from build123d import *

# Parameters (mm, degrees)
SKETCH1_W           = 20
SKETCH1_H           = 16
SKETCH1_R           = 3
SKETCH1_R_2         = 1.5
BOSS_EXTRUDE1_DEPTH = 11.5
CUT_EXTRUDE1_DEPTH  = 17
SKETCH3_R           = 1.5
SKETCH3_R_2         = 0.775
CUT_EXTRUDE2_DEPTH  = 4
CHAMFER1_SIZE       = 0.3


with BuildPart() as part:
    # Sketch1 → Boss-Extrude1 (new body)
    with BuildSketch(Plane(origin=(0, 0, 0), x_dir=(1, 0, 0), z_dir=(0, 1, 0))):
        with Locations((10, 8)):
            Rectangle(SKETCH1_W, SKETCH1_H)
        with Locations((15.5, 8)):
            Circle(SKETCH1_R, mode=Mode.SUBTRACT)
        with Locations((2.5, 8)):
            Circle(SKETCH1_R_2, mode=Mode.SUBTRACT)
    extrude(amount=BOSS_EXTRUDE1_DEPTH)

    # Sketch2 → Cut-Extrude1 (cut, through all)
    with BuildSketch(Plane.XY):
        with BuildLine():
            Line((5.516608474, 4.5), (11.483391526, 4.5))
            ThreePointArc((11.483391526, 4.5), (8.5, 7.025), (5.516608474, 4.5))
        make_face()
        with BuildLine():
            Line((5.516608474, 3.5), (11.483391526, 3.5))
            ThreePointArc((11.483391526, 3.5), (11.514579935, 3.749135861), (11.525, 4))
            ThreePointArc((11.525, 4), (11.514579935, 4.250864139), (11.483391526, 4.5))
            Line((11.483391526, 4.5), (5.516608474, 4.5))
            ThreePointArc((5.516608474, 4.5), (5.475, 4), (5.516608474, 3.5))
        make_face()
        with BuildLine():
            ThreePointArc((5.516608474, 3.5), (8.5, 0.975), (11.483391526, 3.5))
            Line((11.483391526, 3.5), (5.516608474, 3.5))
        make_face()
        with BuildLine():
            Line((0, 3.5), (5.516608474, 3.5))
            ThreePointArc((5.516608474, 3.5), (5.475, 4), (5.516608474, 4.5))
            Line((5.516608474, 4.5), (0, 4.5))
            Line((0, 4.5), (0, 3.5))
        make_face()
    extrude(amount=-CUT_EXTRUDE1_DEPTH, mode=Mode.SUBTRACT)

    # Sketch3 → Cut-Extrude2 (cut)
    with BuildSketch(Plane.XY):
        with Locations((16.5, 4.8)):
            Circle(SKETCH3_R)
        with Locations((18, 2)):
            Circle(SKETCH3_R_2)
    extrude(amount=-CUT_EXTRUDE2_DEPTH, mode=Mode.SUBTRACT)

    # Chamfer1
    chamfer1_edges = [part.edges().sort_by_distance(p)[0] for p in [
        (20, 11.5, -8),
        (10, 11.5, -16),
        (0, 1.75, -16),
        (0, 1.75, 0),
        (0, 11.5, -8),
        (10, 0, -16),
        (20, 0, -8),
        (10, 0, 0),
        (0, 0, -8),
        (10, 11.5, 0),
        (0, 8, -16),
        (20, 5.75, -16),
        (20, 5.75, 0),
        (0, 8, 0),
    ]]
    chamfer(chamfer1_edges, length=CHAMFER1_SIZE)


solid = part.part
Geometry check sheet. Reference: the model listing, model coordinates, mm. A direction names the side the tool comes from. Give positions to 0.01 mm unless a question says otherwise; leave off trailing zeros. Order: outer loops, then holes, each group sorted by start corner. A loop starts at its lowest first (then second) coordinate and runs counter-clockwise, first axis right, second up. Notation, with made-up numbers: M 42.5,80 L 51.5,80 A21 ccw 51.5,92 Z; hole C -18,76.5 d4. An arc over 180 degrees is marked long. Use a Markdown table: item, result.
Item 1: Section check B-B (z = -8). Record the cut outline in (x, y) (3 decimals).
Answers follow:
| item | result |
|---|---|
| outline | M 0,0.3 L 0.3,0 L 1,0 L 1,3.5 L 0,3.5 Z; M 0,4.5 L 1,4.5 L 1,11.5 L 0.3,11.5 L 0,11.2 Z; M 4,0 L 12.5,0 L 12.5,11.5 L 4,11.5 L 4,4.5 L 5.517,4.5 A3.025 cw long 5.517,3.5 L 4,3.5 Z; M 18.5,0 L 19.7,0 L 20,0.3 L 20,11.2 L 19.7,11.5 L 18.5,11.5 Z |
Item 2: Depth check by flat-ended pin: P1, Ø1.5, axis at x = 16, y = 5, coming from the +Z side; P2, Ø5.5, axis at x = 15.5, z = -8, coming from the +Y side. Enter the tip coordinate at first touch or a pass-through.
Answers follow:
| item | result |
|---|---|
| P1 | stops at z = -4 |
| P2 | passes through |
Item 3: Section check C-C (x = 8.5). Record the cut outline in (y, z) (3 decimals), and give its area (3 significant figures).
Answers follow:
| item | result |
|---|---|
| outline | M 0,-15.7 L 0.3,-16 L 0.975,-16 L 0.975,0 L 0.3,0 L 0,-0.3 Z; M 7.025,-16 L 11.2,-16 L 11.5,-15.7 L 11.5,-0.3 L 11.2,0 L 7.025,0 Z |
| area | 87.0 mm2 |
Item 4: Draft check along Y on faces 4 (the flat face through (10, 0, -8)), 5 (the cylindrical face through (12.5, 5.7, -8.1)), 6 (the flat face through (3, 3.5, -10)), 7 (the cylindrical face through (18.74, 2.23, -1.97)). Enter one of: +Y half, -Y half, draft (parallel to the pull), parting line (faces both ways), or undercut.
Answers follow:
| item | result |
|---|---|
| face 4 | -Y half |
| face 5 | draft |
| face 6 | undercut |
| face 7 | undercut |
Item 5: Section check A-A (y = 1.5). Record the cut outline in (x, z), and give its area (3 significant figures).
Answers follow:
| item | result |
|---|---|
| outline | M 0,-15.7 L 0.3,-16 L 6.8,-16 L 6.8,0 L 0.3,0 L 0,-0.3 Z; M 10.2,-16 L 19.7,-16 L 20,-15.7 L 20,-0.3 L 19.7,0 L 18.59,0 L 18.59,-4 L 17.41,-4 L 17.41,0 L 10.2,0 Z; hole C 2.5,-8 d3; hole C 15.5,-8 d6 |
| area | 225 mm2 |
Item 6: Material ranges on line 1 along Y through (x, z) = (16.5, -1.9); line 2 along Z through (x, y) = (2.5, 8.5); line 3 along X through (y, z) = (2.6, -8), recorded low to high.
Answers follow:
| item | result |
|---|---|
| line 1 | y = 0 to 3.3, 6.3 to 11.5 |
| line 2 | z = -16 to -9.5, -6.5 to 0 |
| line 3 | x = 0 to 1, 4 to 5.82, 11.18 to 12.5, 18.5 to 20 |
Item 7: Section check D-D (z = -2). Record the cut outline in (x, y) (3 decimals), and give its area (3 significant figures).
Answers follow:
| item | result |
|---|---|
| outline | M 0,0.3 L 0.3,0 L 19.7,0 L 20,0.3 L 20,11.2 L 19.7,11.5 L 0.3,11.5 L 0,11.2 L 0,4.5 L 5.517,4.5 A3.025 cw long 5.517,3.5 L 0,3.5 Z; hole C 16.5,4.8 d3; hole C 18,2 d1.55 |
| area | 187 mm2 |
Item 8: Tool access check on faces 1 (the flat face through (3, 4.5, -10)), 2 (the cylindrical face through (2.175, 1.726, -6.536)), 3 (the flat face through (18, 2, -4)). Record the directions out of +Z, -Z, +X, -X, +Y, -Y that give a thin tool (end or side, any length) a straight path to the whole face; none if there is none.
Answers follow:
| item | result |
|---|---|
| face 1 | +Z, -Z, -X |
| face 2 | +Y, -Y |
| face 3 | +Z |
